Part model, mm, in its own coordinate system. Face numbers are marked on the shaded views. A direction names the side the tool comes from. Coordinates: 2 decimals unless noted, no trailing zeros. Order: outer loops, then holes, each group sorted by start corner. A loop starts at its lowest first (then second) coordinate and runs counter-clockwise, first axis right, second up. Notation, with made-up numbers: (-30, 13) - (5, 13) arc R16 cw to (5, 25) - close; hole circle Ø3 at (42, 3.5). An arc over 180 degrees is marked (long way). Use a Markdown table: item, result. Add a question column.
1) Saw through at B-B on y = 8.5. List the corners of the cut face in (x, z), then the cut area to 3 significant figures.
2) Saw through at D-D on y = 16. List the corners of the cut face in (x, z), then the cut area to 3 significant figures.
3) Two-plate mould, pull along X, no slides. Class the marked faces 1, 2 and 3: +X half, -X half, draft (parallel to the pull), parting line (faces both ways), or undercut.
4) Wall check: L1, parallel to Y at x = 54.75, z = 1.65; L2, parallel to Z at x = 4.5, y = 11.5. Give the ranges that are in metal, low to high. Write a range as [from, to].
5) Saw through at C-C on z = 6. List the corners of the cut face in (x, y), then the cut area to 3 significant figures.
6) Tool access for the marked faces 4 and 5: list every direction of +Z, -Z, +X, -X, +Y, -Y with a clear straight run to the whole face (end or side of a thin tool).
7) Drop flat-ended pins along their axis: P1, Ø0.9, axis at y = 2, z = 9.5, coming from the -X side; P2, Ø2, axis at x = 46, y = 5.5, coming from the -Z side; P3, Ø1.9, axis at x = 39, y = 1.5, coming from the +Z side; P4, Ø11, axis at x = 4, y = 8, coming from the +Z side. Give the stop position or say it passes through.
8) Saw through at A-A on x = 6.65. List the corners of the cut face in (y, z), then the cut area to 3 significant figures.
```python
from build123d import *

# Parameters (mm, degrees)
SKETCH1_R           = 1.5
BOSS_EXTRUDE1_DEPTH = 3
SKETCH2_W           = 10
SKETCH2_H           = 3
BOSS_EXTRUDE2_DEPTH = 10
FILLET1_R           = 2


with BuildPart() as part:
    # Sketch1 → Boss-Extrude1 (new body)
    with BuildSketch(Plane.XY):
        Polygon((10, 24), (10, 3), (51.4, 3), (51.4, 24), (61.4, 24), (61.4, 0), (0, 0), (0, 24), align=None)
        with Locations((6.65, 8.5)):
            Circle(SKETCH1_R, mode=Mode.SUBTRACT)
        with Locations((6.65, 18.5)):
            Circle(SKETCH1_R, mode=Mode.SUBTRACT)
        with Locations((54.75, 18.5)):
            Circle(SKETCH1_R, mode=Mode.SUBTRACT)
        with Locations((54.75, 8.5)):
            Circle(SKETCH1_R, mode=Mode.SUBTRACT)
    extrude(amount=BOSS_EXTRUDE1_DEPTH)

    # Sketch2 → Boss-Extrude2 (add)
    with BuildSketch(Plane.XY.offset(3)):
        with Locations((15, 1.5)):
            Rectangle(SKETCH2_W, SKETCH2_H)
        with Locations((46.4, 1.5)):
            Rectangle(SKETCH2_W, SKETCH2_H)
        with Locations((30.7, 1.5)):
            Rectangle(SKETCH2_W, SKETCH2_H)
    extrude(amount=BOSS_EXTRUDE2_DEPTH)

    # Fillet1
    fillet1_edges = [part.edges().sort_by_distance(p)[0] for p in [
        (10, 1.5, 3),
        (51.4, 1.5, 3),
        (20, 1.5, 3),
        (10, 1.5, 13),
        (20, 1.5, 13),
        (25.7, 1.5, 3),
        (41.4, 1.5, 3),
        (35.7, 1.5, 3),
        (25.7, 1.5, 13),
        (35.7, 1.5, 13),
        (41.4, 1.5, 13),
        (51.4, 1.5, 13),
        (51.4, 24, 1.5),
        (61.4, 24, 1.5),
        (61.4, 0, 1.5),
        (0, 0, 1.5),
        (0, 24, 1.5),
        (10, 24, 1.5),
    ]]
    fillet(fillet1_edges, radius=FILLET1_R)


solid = part.part
```
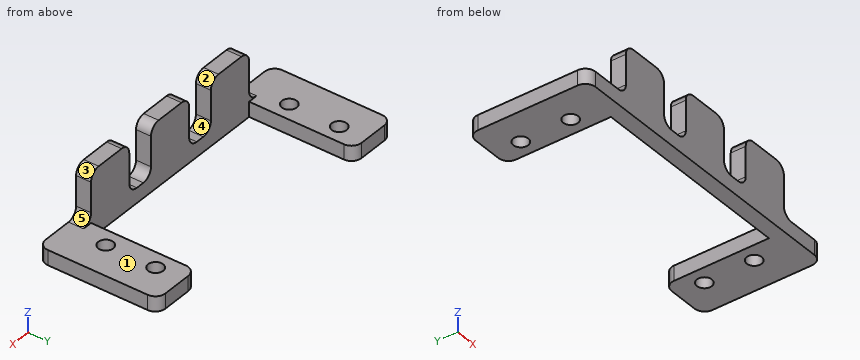
Results are:
| question | item | result |
|---|---|---|
| 1 | outline | (0, 0) - (5.15, 0) - (5.15, 3) - (0, 3) - close; (8.15, 0) - (10, 0) - (10, 3) - (8.15, 3) - close; (51.4, 0) - (53.25, 0) - (53.25, 3) - (51.4, 3) - close; (56.25, 0) - (61.4, 0) - (61.4, 3) - (56.25, 3) - close |
| 1 | area | 42.0 mm2 |
| 2 | outline | (0, 0) - (10, 0) - (10, 3) - (0, 3) - close; (51.4, 0) - (61.4, 0) - (61.4, 3) - (51.4, 3) - close |
| 2 | area | 60.0 mm2 |
| 3 | face 1 | draft |
| 3 | face 2 | undercut |
| 3 | face 3 | +X half |
| 4 | L1 | [0, 7], [10, 17], [20, 24] |
| 4 | L2 | [0, 3] |
| 5 | outline | (10, 0) - (20, 0) - (20, 3) - (10, 3) - close; (25.7, 0) - (35.7, 0) - (35.7, 3) - (25.7, 3) - close; (41.4, 0) - (51.4, 0) - (51.4, 3) - (41.4, 3) - close |
| 5 | area | 90.0 mm2 |
| 6 | face 4 | +Z, +Y, -Y |
| 6 | face 5 | +Z, +X, +Y, -Y |
| 7 | P1 | x = 10 |
| 7 | P2 | through |
| 7 | P3 | z = 3.08 |
| 7 | P4 | z = 3 |
| 8 | outline | (0, 0) - (7, 0) - (7, 3) - (0, 3) - close; (10, 0) - (17, 0) - (17, 3) - (10, 3) - close; (20, 0) - (24, 0) - (24, 3) - (20, 3) - close |
| 8 | area | 54.0 mm2 |
